from build123d import *

# Parameters (mm, degrees)
SKETCH1_W           = 25
SKETCH1_H           = 25
BOSS_EXTRUDE1_DEPTH = 90
SKETCH2_R           = 4.05
CUT_EXTRUDE1_DEPTH  = 8
SKETCH3_R           = 4.05
CUT_EXTRUDE7_DEPTH  = 8
CHAMFER1_SIZE       = 2
SKETCH5_R           = 1.6
CUT_EXTRUDE8_DEPTH  = 12.5
SKETCH7_R           = 1.6
CUT_EXTRUDE9_DEPTH  = 10


with BuildPart() as part:
    # Sketch1 → Boss-Extrude1 (new body)
    with BuildSketch(Plane(origin=(0, 0, 0), x_dir=(1, 0, 0), z_dir=(0, 1, 0))):
        Rectangle(SKETCH1_W, SKETCH1_H)
    extrude(amount=BOSS_EXTRUDE1_DEPTH)

    # Sketch2 → Cut-Extrude1 (cut)
    with BuildSketch(Plane(origin=(12.5, 0, 0), x_dir=(0, 0, -1), z_dir=(1, 0, 0))):
        with Locations((0, 71)):
            Circle(SKETCH2_R)
        with Locations((0, 29)):
            Circle(SKETCH2_R)
    extrude(amount=-CUT_EXTRUDE1_DEPTH, mode=Mode.SUBTRACT)

    # Sketch3 → Cut-Extrude7 (cut)
    with BuildSketch(Plane.XY.offset(12.5)):
        with Locations((0, 29)):
            Circle(SKETCH3_R)
        with Locations((0, 71)):
            Circle(SKETCH3_R)
    extrude(amount=-CUT_EXTRUDE7_DEPTH, mode=Mode.SUBTRACT)

    # Chamfer1
    chamfer1_edges = [part.edges().sort_by_distance(p)[0] for p in [
        (12.5, 45, 12.5),
        (-12.5, 45, 12.5),
        (-12.5, 45, -12.5),
        (12.5, 45, -12.5),
    ]]
    chamfer(chamfer1_edges, length=CHAMFER1_SIZE)

    # Sketch5 → Cut-Extrude8 (cut)
    with BuildSketch(Plane(origin=(12.5, 0, 0), x_dir=(0, 0, -1), z_dir=(1, 0, 0))):
        with Locations((0, 59)):
            Circle(SKETCH5_R)
        with Locations((0, 41)):
            Circle(SKETCH5_R)
    extrude(amount=-CUT_EXTRUDE8_DEPTH, mode=Mode.SUBTRACT)

    # Sketch7 → Cut-Extrude9 (cut)
    with BuildSketch(Plane(origin=(0, 90, 0), x_dir=(1, 0, 0), z_dir=(0, 1, 0))):
        Circle(SKETCH7_R)
    extrude(amount=-CUT_EXTRUDE9_DEPTH, mode=Mode.SUBTRACT)


solid = part.part
Geometry check sheet. Reference: the model listing, model coordinates, mm. A direction names the side the tool comes from. Coordinates: 2 decimals unless noted, no trailing zeros. Order: outer loops, then holes, each group sorted by start corner. A loop starts at its lowest first (then second) coordinate and runs counter-clockwise, first axis right, second up. Notation, with made-up numbers: (-33.5, 16) - (-19.5, 16) arc R14 cw to (-19.5, 28) - close; hole circle Ø2 at (-36, 56.25). An arc over 180 degrees is marked (long way). Answer in a Markdown table with one row per item. Add a question column.
1) Set-up check for faces 4 (the flat face through (0, 0, 0)), 5 (the cylindrical face through (6.338, 60.586, 0.208)), 6 (the cylindrical face through (-1.27, 85.07, 0.97)), 7 (the cylindrical face through (2.2, 74.4, 8.6)): record each of +Z, -Z, +X, -X, +Y, -Y from which the full face is reachable in a straight line by a thin tool's end or side.
2) Release check for a two-part mould opening along Z. For faces 1 (the cylindrical face through (-0.878, 25.046, 8.556)), 2 (the flat face through (0, 80, 0)), 3 (the flat face through (0, 71, 4.5)) record: +Z half, -Z half, draft (parallel to the pull), parting line (faces both ways), or undercut.
3) Gauge pin test, flat ends, axial feed: P1, Ø2.5, axis at x = 0, y = 28, coming from the +Z side; P2, Ø2.5, axis at y = 71, z = -1, coming from the +X side; P3, Ø1, axis at y = 41.5, z = -0.5, coming from the +X side. Record the tip position at first contact, or that the pin passes through.
4) Material ranges on line 1 along Y through (x, z) = (0.5, 10); line 2 along Y through (x, z) = (10.25, 0); line 3 along Y through (x, z) = (1.25, -1.25), recorded low to high. Write a range as [from, to].
5) Cross-section at D-D, the plane z = 0. Record the cut outline in (x, y), then the cut area to 3 significant figures.
6) Cross-section at B-B, the plane z = 6.5. Record the cut outline in (x, y), then the cut area to 3 significant figures.
7) Cross-section at C-C, the plane y = 41. Record the cut outline in (x, z).
8) Cross-section at A-A, the plane y = 82.5. Record the cut outline in (x, z).
Check result:
| question | item | result |
|---|---|---|
| 1 | face 4 | +Z, -Z, +X, -X, -Y |
| 1 | face 5 | +X |
| 1 | face 6 | +Y |
| 1 | face 7 | +Z |
| 2 | face 1 | draft |
| 2 | face 2 | undercut |
| 2 | face 3 | +Z half |
| 3 | P1 | stops at z = 4.5 |
| 3 | P2 | stops at x = 4.5 |
| 3 | P3 | stops at x = 0 |
| 4 | line 1 | y = [0, 24.98], [33.02, 66.98], [75.02, 90] |
| 4 | line 2 | y = [0, 24.95], [33.05, 39.4], [42.6, 57.4], [60.6, 66.95], [75.05, 90] |
| 4 | line 3 | y = [0, 40], [42, 58], [60, 90] |
| 5 | outline | (-12.5, 0) - (12.5, 0) - (12.5, 24.95) - (4.5, 24.95) - (4.5, 33.05) - (12.5, 33.05) - (12.5, 39.4) - (0, 39.4) - (0, 42.6) - (12.5, 42.6) - (12.5, 57.4) - (0, 57.4) - (0, 60.6) - (12.5, 60.6) - (12.5, 66.95) - (4.5, 66.95) - (4.5, 75.05) - (12.5, 75.05) - (12.5, 90) - (1.6, 90) - (1.6, 80) - (-1.6, 80) - (-1.6, 90) - (-12.5, 90) - close |
| 5 | area | 2,010 mm² |
| 6 | outline | (-12.5, 0) - (12.5, 0) - (12.5, 90) - (-12.5, 90) - close; hole circle Ø8.1 at (0, 29); hole circle Ø8.1 at (0, 71) |
| 6 | area | 2,150 mm² |
| 7 | outline | (-12.5, -10.5) - (-10.5, -12.5) - (10.5, -12.5) - (12.5, -10.5) - (12.5, -1.6) - (0, -1.6) - (0, 1.6) - (12.5, 1.6) - (12.5, 10.5) - (10.5, 12.5) - (-10.5, 12.5) - (-12.5, 10.5) - close |
| 8 | outline | (-12.5, -10.5) - (-10.5, -12.5) - (10.5, -12.5) - (12.5, -10.5) - (12.5, 10.5) - (10.5, 12.5) - (-10.5, 12.5) - (-12.5, 10.5) - close; hole circle Ø3.2 at (0, 0) |
